Input: part model. Units: mm. Frame: model coordinates. Face numbers are marked on the shaded views. A direction names the side the tool comes from. Round coordinates to 2 decimals unless told otherwise and drop trailing zeros. Order: outer loops, then holes, each group sorted by start corner. A loop starts at its lowest first (then second) coordinate and runs counter-clockwise, first axis right, second up. Notation, with made-up numbers: (47.25, 41) -> (55.25, 41) arc R21 ccw to (55.25, 62) -> close; hole circle Ø10 at (76.25, 58). An arc over 180 degrees is marked (long way). Answer as CSV lines item,"result". Start each with the question number.
1) First-contact query: P1, Ø6.5, axis at x = 49.5, y = 41, coming from the +Z side; P2, Ø3.5, axis at x = 78.5, y = 9, coming from the -Z side. Flat tips, straight axial feed; report the tip coordinate or a pass-through.
2) Section query A-A, the plane y = 42.85. Output: boundary loops of the cut face in (x, z).
3) Access query for the marked faces 5, 6 and 7. Directions: +Z, -Z, +X, -X, +Y, -Y. A direction counts if a zero-diameter tool reaches every point of the face in a straight line with its end or side. Return the directions, or none.
4) Section query C-C, the plane x = 50. Output: boundary loops of the cut face in (y, z), and give its area (3 significant figures).
5) Line query: L1, parallel to X at y = 10, z = 2.25; L2, parallel to Y at x = 40, z = 9.5; L3, parallel to Y at x = 60, z = 3. Output: solid intervals per line, ascending.
6) Section query B-B, the plane x = 80. Output: boundary loops of the cut face in (y, z).
7) Mould query, pull axis Y, two halves, no side actions, for the marked faces 1, 2, 3 and 4. Classes: +Y half, -Y half, draft (parallel to the pull), parting line (faces both ways), or undercut.
8) Section query D-D, the plane z = 9.25. Output: boundary loops of the cut face in (x, y).
```python
from build123d import *

# Parameters (mm, degrees)
SKETCH_W        = 100
SKETCH_H        = 64
SKETCH_R        = 5
SKETCH_R_2      = 3.2
SKETCH_R_3      = 4
PAD_DEPTH       = 15
SKETCH001_R     = 11.02
POCKET_DEPTH    = 7.2
SKETCH002_R     = 6
POCKET001_DEPTH = 7
SKETCH003_R     = 3.2
POCKET002_DEPTH = 15


with BuildPart() as part:
    # Sketch → Pad (new body)
    with BuildSketch(Plane.XY):
        with Locations((50, 32)):
            Rectangle(SKETCH_W, SKETCH_H)
        with Locations((50, 42.85)):
            Circle(SKETCH_R, mode=Mode.SUBTRACT)
        with Locations((20, 10)):
            Circle(SKETCH_R_2, mode=Mode.SUBTRACT)
        with Locations((80, 10)):
            Circle(SKETCH_R_2, mode=Mode.SUBTRACT)
        with Locations((82, 42.85)):
            Circle(SKETCH_R_3, mode=Mode.SUBTRACT)
        with Locations((18, 42.85)):
            Circle(SKETCH_R_3, mode=Mode.SUBTRACT)
    extrude(amount=PAD_DEPTH)

    # Sketch001 (on Face11 of Pad) → Pocket (cut)
    with BuildSketch(Plane.XY.offset(15)):
        with Locations((50, 42.85)):
            Circle(SKETCH001_R)
    extrude(amount=-POCKET_DEPTH, mode=Mode.SUBTRACT)

    # Sketch002 (on Face4 of Pocket) → Pocket001 (cut)
    with BuildSketch(Plane(origin=(0, 0, 0), x_dir=(1, 0, 0), z_dir=(0, 0, -1))):
        with Locations((20, -10)):
            Circle(SKETCH002_R)
        with Locations((80, -10)):
            Circle(SKETCH002_R)
        with Locations((40, -10)):
            Circle(SKETCH002_R)
        with Locations((60, -10)):
            Circle(SKETCH002_R)
    extrude(amount=-POCKET001_DEPTH, mode=Mode.SUBTRACT)

    # Sketch003 (on Face5 of Pocket001) → Pocket002 (cut)
    with BuildSketch(Plane.XY.offset(15)):
        with Locations((40, 10)):
            Circle(SKETCH003_R)
        with Locations((60, 10)):
            Circle(SKETCH003_R)
    extrude(amount=-POCKET002_DEPTH, mode=Mode.SUBTRACT)


solid = part.part
```
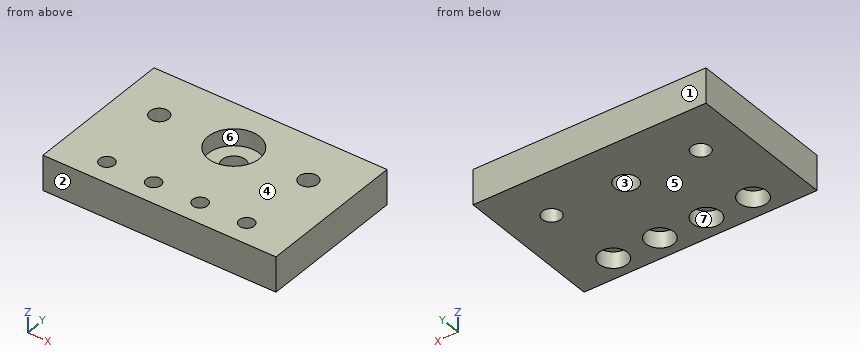
Findings:
1,P1,"stops at z = 7.8"
1,P2,"stops at z = 7"
2,outline,"(0, 0) -> (14, 0) -> (14, 15) -> (0, 15) -> close; (22, 0) -> (45, 0) -> (45, 7.8) -> (38.98, 7.8) -> (38.98, 15) -> (22, 15) -> close; (55, 0) -> (78, 0) -> (78, 15) -> (61.02, 15) -> (61.02, 7.8) -> (55, 7.8) -> close; (86, 0) -> (100, 0) -> (100, 15) -> (86, 15) -> close"
3,face 5,"-Z, +X, -X, +Y, -Y"
3,face 6,"+Z"
3,face 7,"-Z"
4,outline,"(0, 0) -> (37.85, 0) -> (37.85, 7.8) -> (31.83, 7.8) -> (31.83, 15) -> (0, 15) -> close; (47.85, 0) -> (64, 0) -> (64, 15) -> (53.87, 15) -> (53.87, 7.8) -> (47.85, 7.8) -> close"
4,area,"723 mm^2"
5,L1,"x = 0 to 14, 26 to 34, 46 to 54, 66 to 74, 86 to 100"
5,L2,"y = 0 to 6.8, 13.2 to 38.22, 47.48 to 64"
5,L3,"y = 0 to 4, 16 to 64"
6,outline,"(0, 0) -> (4, 0) -> (4, 7) -> (6.8, 7) -> (6.8, 15) -> (0, 15) -> close; (13.2, 7) -> (16, 7) -> (16, 0) -> (39.39, 0) -> (39.39, 15) -> (13.2, 15) -> close; (46.31, 0) -> (64, 0) -> (64, 15) -> (46.31, 15) -> close"
7,face 1,"+Y half"
7,face 2,"-Y half"
7,face 3,"undercut"
7,face 4,"draft"
8,outline,"(0, 0) -> (100, 0) -> (100, 64) -> (0, 64) -> close; hole circle Ø8 at (18, 42.85); hole circle Ø6.4 at (20, 10); hole circle Ø6.4 at (40, 10); hole circle Ø22.04 at (50, 42.85); hole circle Ø6.4 at (60, 10); hole circle Ø6.4 at (80, 10); hole circle Ø8 at (82, 42.85)"
